Autodesk Inventor part; units mm, degrees
ref_plane "MSC_PF1" through (0, 0, 0) normal (1, 0, 0) x (0, 1, 0)
ref_plane "MSC_PT1" through (0, 0, 0) normal (0, 0, -1) x (-1, 0, 0)
ref_plane "YZ Plane" through (0, 0, 0) normal (1, 0, 0) x (0, 1, 0)
sketch "Эскиз2" plane through (0, 0, 0) normal (0, 0, 1) x (1, 0, 0)
  circle A0 centre (0, 0) radius 1.25
  dimension "d3" = 2.5
extrude "Выдавливание1" add sketch "Эскиз2" against normal blind 0.94
sketch "Эскиз3" plane through (0, 0, -0.94) normal (0, 0, -1) x (-1, 0, 0)
  circle A0 centre (0, 0) radius 1.5
  circle A1 centre (0, 0) radius 1.25 construction
  dimension "d28" = 360
  dimension "d9" = 3
extrude "Выдавливание2" add sketch "Эскиз3" along normal blind 5.06
chamfer "Фаска1" distance 0.25 distance2 0.25 1 edges at (1.5, 0, -0.94) measured on face at (-1.39, -0.2194, -0.94)
sketch "Эскиз4" plane through (0, 0, 0) normal (0, 0, 1) x (1, 0, 0)
  circle A0 centre (0, 0) radius 3.15
  circle A1 centre (0, 0) radius 1.25 construction
  dimension "d15" = 6.3
extrude "Выдавливание3" add sketch "Эскиз4" along normal blind 1.3
fillet "Сопряжение1" radius 0.1 1 edges at (-1.25, 0, 0)
sketch "Эскиз5" plane through (0, 0, 0) normal (0, 1, 0) x (-1, 0, 0)
  line L0 (3.15, 1.3) -> (3.15, 0)
  line L1 (3.0363, 1.3) -> (3.15, 1.3)
  line L2 (3.15, 0) -> (3.0363, 1.3)
  line L3 (-3.15, 1.3) -> (3.15, 1.3) construction
  line L4 (-3.15, 0) -> (3.15, 0) construction
  line L5 (0, -0.26) -> (0, 1.56)
  line L6 (4.41, 0) -> (-4.41, 0)
  dimension "d20" = 5
  dimension "d56" = 3.15
  dimension "d57" = 1.3
revolve "Вращение1" cut sketch "Эскиз5" angle 360 about axis through (0, 0, -10) along (0, 0, 1)
sketch "Эскиз6" plane through (0, 0, 0) normal (0, 1, 0) x (-1, 0, 0)
  line L0 (0, 1.9) -> (0, 1.3)
  arc A0 (3.0363, 1.3) -> (0, 1.9) centre (-0.906, -10.6674) ccw
  line L1 (0, 1.3) -> (3.0363, 1.3)
  line L2 (3.0363, 1.3) -> (-3.0363, 1.3) construction
  line L3 (0, -4.4495) -> (0, 0.4495)
  line L4 (0, -13.1996) -> (0, 4.5258)
  line L5 (4.273, 0) -> (-4.2545, 0)
  dimension "d58" = 0.6
  dimension "d59" = 3.0363
  dimension "d60" = 0
  dimension "d62" = 12.6
revolve "Вращение2" add sketch "Эскиз6" angle 360 about axis through (0, 0, -4.4495) along (0, 0, 1)
sketch "Эскиз7" plane through (0, 0, 0) normal (0, 1, 0) x (-1, 0, 0)
  line L0 (1.85, 1.9) -> (-1.85, 1.9)
  line L1 (1.1365, 0.37) -> (1.85, 1.9)
  line L2 (-1.1365, 0.37) -> (1.1365, 0.37)
  line L3 (-1.85, 1.9) -> (-1.1365, 0.37)
  line L4 (0, 0.064) -> (0, 2.206)
  line L5 (2.59, 0) -> (-2.59, 0)
  dimension "d32" = 1.53
  dimension "d34" = 65
  dimension "d36" = 65
  dimension "d63" = 1.85
  dimension "d64" = 1.9
  dimension "d65" = 3.7
extrude "Выдавливание4" cut sketch "Эскиз7" against normal mid plane 1.2333
sketch "Эскиз8" plane through (0, 0, 0) normal (1, 0, 0) x (0, 1, 0)
  line L0 (-1.1365, 0.37) -> (-1.85, 1.9)
  line L1 (1.1365, 0.37) -> (-1.1365, 0.37)
  line L2 (1.85, 1.9) -> (1.1365, 0.37)
  line L3 (-1.85, 1.9) -> (1.85, 1.9)
  line L4 (0, 0.064) -> (0, 2.206)
  line L5 (-2.59, 0) -> (2.59, 0)
  dimension "d40" = 65
  dimension "d42" = 65
  dimension "d44" = 1.53
  dimension "d66" = 3.7
  dimension "d67" = 1.9
  dimension "d69" = 1.85
extrude "Выдавливание5" cut sketch "Эскиз8" along normal mid plane 1.2333
sketch "Эскиз9" plane through (0, 0, 0) normal (0, 1, 0) x (-1, 0, 0)
  line L0 (0, 1.9) -> (0, 0.37)
  line L1 (1.48, 1.9) -> (0, 1.9)
  line L2 (0, 0.37) -> (1.48, 1.9)
  line L3 (-3.15, 0) -> (3.15, 0) construction
  line L4 (0, -0.38) -> (0, 2.28)
  line L5 (4.41, 0) -> (-4.41, 0)
  dimension "d50" = 1.53
  dimension "d52" = 1.53
  dimension "d54" = 1.48
  dimension "d70" = 0
  dimension "d71" = 1.9
revolve "Вращение3" cut sketch "Эскиз9" angle 360 about axis through (0, 0, -10) along (0, 0, 1)
thread "Резьба1"
ref_plane "MSC_PF1" through (0, 0, 0) normal (1, 0, 0) x (0, 1, 0)
ref_plane "MSC_PT1" through (0, 0, 0) normal (0, 0, -1) x (-1, 0, 0)
equation "\"d4\" = -b + NLG"
equation "\"d9\" = NND"
equation "\"d10\" = b"
equation "\"d12\" = -0.5 * msp_ds + 0.5 * NND"
equation "\"d13\" = 0.5 * NND - 0.5 * msp_ds"
equation "\"d15\" = Dk"
equation "\"d16\" = ParK"
equation "\"d18\" = r"
equation "\"d32\" = q"
equation "\"d63\" = 0.5 * M"
equation "\"d64\" = ParK + ParF"
equation "\"d65\" = M"
equation "\"d37\" = 2 * msp_s"
equation "\"d44\" = q"
equation "\"d66\" = M"
equation "\"d67\" = ParK + ParF"
equation "\"d69\" = 0.5 * M"
equation "\"d47\" = 2 * msp_s"
equation "\"d3\" = msp_ds"
equation "\"d56\" = 0.5 * Dk"
equation "\"d57\" = ParK"
equation "\"d58\" = ParF"
equation "\"d59\" = 0.5 * Dk - msp_v"
equation "\"d62\" = 2 * Dk"
equation "\"d50\" = q"
equation "\"d52\" = q"
equation "\"d54\" = msp_rr"
equation "\"d71\" = ParK + ParF"
equation "\"PTC\" = 0.5"
equation "\"NLG\" = 6"
equation "\"Dk\" = 6.3"
equation "\"ParK\" = 1.3"
equation "\"NND\" = 3"
equation "\"M\" = 3.7"
equation "\"q\" = 1.53"
equation "\"r\" = 0.1"
equation "\"msp_ds\" = NND - PTC"
equation "\"b\" = 5.06"
equation "\"msp_x\" = 1.25 * PTC"
equation "\"msp_s\" = 0.166667 * M"
equation "\"msp_rr\" = 0.4 * M"
equation "\"ParF\" = 0.6"
equation "\"msp_v\" = 0.0874887 * ParK"
equation "\"THREADDIA\" = NND"
properties part number "JIS B 1111 - M3x6" material "Сталь, мягкая"
Check sheet for the modelled part. Datum: model origin and axes. Units: mm. A direction names the side the tool comes from. Give positions to 0.01 mm unless a question says otherwise; leave off trailing zeros. Order: outer loops, then holes, each group sorted by start corner. A loop starts at its lowest first (then second) coordinate and runs counter-clockwise, first axis right, second up. Notation, with made-up numbers: M 19.25,-9 L 55.25,-9 A21 ccw 55.25,28 Z; hole C 62.25,4 d5. An arc over 180 degrees is marked long. Answer as CSV lines item,"result". Start each with the question number.
Item 1: Cross-section at A-A on z = -2. Enter the section's corners in (x, y), plus the area to 3 significant figures.
Item 2: Mould release check, pull along Y, two halves, no side actions. Record for faces 3 (the face through (-0.617, 1, 1)), 4 (the face through (0, 0, -6)), 5 (the face through (1.5, -0.07, -3.56)): +Y half, -Y half, draft (parallel to the pull), parting line (faces both ways), or undercut.
Item 3: Gauge pin test, flat ends, axial feed: P1, Ø3, axis at x = 1, z = -2, coming from the +Y side; P2, Ø1.2, axis at y = 1.5, z = 1, coming from the +X side; P3, Ø0.6, axis at x = 1.5, z = 1.5, coming from the +Y side (3 decimals). Record the tip position at first contact, or that the pin passes through.
Item 4: Tool access check on faces 1 (the face through (1.44, 0.01, 1.02)), 2 (the face through (-0.27, -1.22, -0.51)). Record the directions out of +Z, -Z, +X, -X, +Y, -Y that give a thin tool (end or side, any length) a straight path to the whole face; none if there is none.
Item 5: Thickness scan on line 1 (Y direction, x = 0, z = -0.5); line 2 (Z direction, x = 0.5, y = -0.75); line 3 (Y direction, x = 0, z = 0.5). Record the ranges inside material, lowest first. Write a range as [from, to].
Established:
1,outline,"C 0,0 d3"
1,area,"7.07 mm^2"
2,face 3,"undercut"
2,face 4,"draft"
2,face 5,"parting line"
3,P1,"stops at y = 1.5"
3,P2,"stops at x = 2.94"
3,P3,"stops at y = 2.755"
4,face 1,"+Z"
4,face 2,"none"
5,line 1,"y = [-1.25, 1.25]"
5,line 2,"z = [-6, 0.37]"
5,line 3,"y = [-3.11, -1.2], [1.2, 3.11]"
